Work out the finished part from the listing and answer in its coordinate system (mm). Coordinates: 2 decimals unless noted, no trailing zeros. Write each loop counter-clockwise with the first axis right and the second up, starting at its lowest first coordinate (ties: lowest second). Pieces come first, ordered by that corner, then holes. Notation, with made-up numbers: (19.5, 67.5) -> (35.5, 67.5) arc R11 ccw to (35.5, 84.5) -> close; hole circle Ø8 at (-14, -14.5). An arc over 180 degrees is marked (long way). Write each question's results on one line, items separated by ' | '. Start each with the question number.
from build123d import *

# Parameters (mm, degrees)
F1_DEPTH = 19.05
F2_R     = 6.35
F3_DEPTH = 19.051


with BuildPart() as f1:
    # F0 (on Right) → F1 (new body)
    with BuildSketch(Plane.YZ):
        with BuildLine():
            ThreePointArc((-254, 0), (-159.564589, -136.006104), (-7.957927, -202.572815))
            ThreePointArc((-7.957927, -202.572815), (26.7802, -195.567823), (48.486376, -167.556231))
            ThreePointArc((48.486376, -167.556231), (117.175368, -68.177885), (230.136876, -25.353462))
            ThreePointArc((230.136876, -25.353462), (247.0959, -17.408667), (254, 0))
            Line((254, 0), (-254, 0))
        make_face()
    extrude(amount=F1_DEPTH)

    # F2 (on face) → F3 (cut, through all)
    with BuildSketch(Plane.YZ.offset(19.05)):
        with Locations((0, -177.8)):
            Circle(F2_R)
        with Locations((0, -76.2)):
            Circle(F2_R)
    extrude(amount=-F3_DEPTH, mode=Mode.SUBTRACT)


solid = f1.part
1. Find section B-B on x = 6.5. Give the vertices of the cut face in (y, z).
2. Find the intervals of material crossed by L1, parallel to Z at x = 7, y = 0; L2, parallel to Y at x = 13.5, z = -64; L3, parallel to Y at x = 17, z = -88, in increasing order.
3. Given pin 1 Ø11.5 at (y, z) = (0, -76.2) entering from -X; pin 2 Ø3 at (x, z) = (16, -159) entering from -Y; pin 3 Ø5 at (x, z) = (10, -94.5) entering from +Y; pin 4 Ø16.5 at (y, z) = (0, -177.8) entering from +X, each flat-ended and moving along its own axis, determine where each tip first touches the part or whether it passes through.
4. Find section A-A on y = 0. Give the vertices of the cut face in (x, z).
5. Find section C-C on z = -76.2. Give the vertices of the cut face in (x, y), and give its area (3 significant figures).
6. Determine the mould class of faces 1 (the face through (9.658, 3.414, -70.846)), 2 (the face through (9.39, -161.37, -134.51)), 3 (the face through (0, -60, -78)) for opening direction Y: pulls with the +Y half, pulls with the -Y half, needs draft (parallel to the pull), parting line crosses it, or undercut.
7. Find section D-D on z = -177.8. Give the vertices of the cut face in (x, y).
Ans:
1) outline: (-254, 0) arc R304.8 ccw to (-7.96, -202.57) arc R50.8 ccw to (48.49, -167.56) arc R203.2 cw to (230.14, -25.35) arc R25.4 ccw to (254, 0) -> close; hole circle Ø12.7 at (0, -177.8); hole circle Ø12.7 at (0, -76.2)
2) L1: z = -203.2 to -184.15, -171.45 to -82.55, -69.85 to 0 | L2: y = -223.19 to 122.7 | L3: y = -206.29 to 95.33
3) pin 1: passes through | pin 2: stops at y = -130.01 | pin 3: stops at y = 91.62 | pin 4: stops at x = 19.05
4) outline: (0, -203.2) -> (19.05, -203.2) -> (19.05, -184.15) -> (0, -184.15) -> close; (0, -171.45) -> (19.05, -171.45) -> (19.05, -82.55) -> (0, -82.55) -> close; (0, -69.85) -> (19.05, -69.85) -> (19.05, 0) -> (0, 0) -> close
5) outline: (0, -215.03) -> (19.05, -215.03) -> (19.05, -6.35) -> (0, -6.35) -> close; (0, 6.35) -> (19.05, 6.35) -> (19.05, 107.55) -> (0, 107.55) -> close | area: 5,900 mm²
6) face 1: undercut | face 2: pulls with the -Y half | face 3: needs draft
7) outline: (0, -92.78) -> (19.05, -92.78) -> (19.05, -6.35) -> (0, -6.35) -> close; (0, 6.35) -> (19.05, 6.35) -> (19.05, 43.99) -> (0, 43.99) -> close
